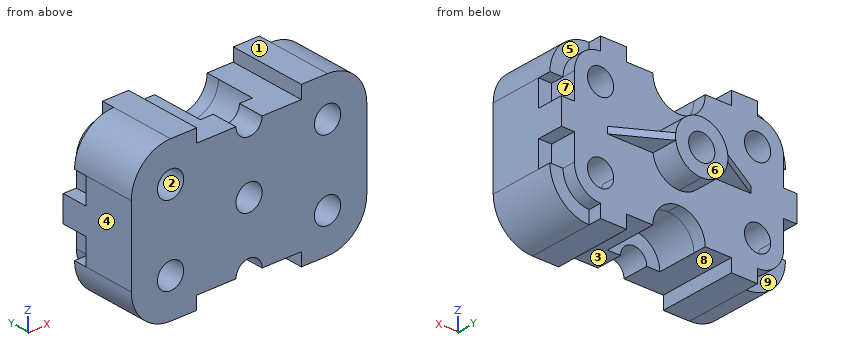
```python
from build123d import *

# Parameters (mm, degrees)
SKETCH1_W           = 180
SKETCH1_H           = 120
BOSS_EXTRUDE2_DEPTH = 80
CUT_EXTRUDE1_DEPTH  = 150
CUT_EXTRUDE2_DEPTH  = 150
SKETCH4_R           = 10
CUT_EXTRUDE3_DEPTH  = 150
CUT_EXTRUDE4_DEPTH  = 60
CUT_EXTRUDE5_DEPTH  = 60
SKETCH7_R           = 10
CUT_EXTRUDE7_DEPTH  = 139
SKETCH8_W           = 80
SKETCH8_H           = 10
CUT_EXTRUDE8_DEPTH  = 139
BOSS_EXTRUDE3_DEPTH = 60
CUT_EXTRUDE9_DEPTH  = 256
CUT_EXTRUDE10_DEPTH = 60
CUT_EXTRUDE11_DEPTH = 60
SKETCH13_W          = 40
SKETCH13_H          = 20
SKETCH13_W_2        = 20
SKETCH13_H_2        = 10
CUT_EXTRUDE12_DEPTH = 209
CUT_EXTRUDE13_DEPTH = 20
CUT_EXTRUDE14_DEPTH = 10
CUT_EXTRUDE15_DEPTH = 10
CUT_EXTRUDE16_DEPTH = 10
CUT_EXTRUDE17_DEPTH = 10
BOSS_EXTRUDE4_DEPTH = 10
BOSS_EXTRUDE5_DEPTH = 10
SKETCH21_W          = 10
SKETCH21_H          = 20
CUT_EXTRUDE20_DEPTH = 20
SKETCH22_W          = 35
SKETCH22_H          = 5
BOSS_EXTRUDE9_DEPTH = 19.999
CUT_EXTRUDE21_DEPTH = 10


with BuildPart() as part:
    # Sketch1 → Boss-Extrude2 (new body)
    with BuildSketch(Plane(origin=(0, 0, 0), x_dir=(1, 0, 0), z_dir=(0, 1, 0))):
        with Locations((90, 60)):
            Rectangle(SKETCH1_W, SKETCH1_H)
    extrude(amount=BOSS_EXTRUDE2_DEPTH)

    # Sketch2 → Cut-Extrude1 (cut)
    with BuildSketch(Plane(origin=(0, 0, 0), x_dir=(1, 0, 0), z_dir=(0, 1, 0))):
        with BuildLine():
            ThreePointArc((30, 0), (8.786796564, 8.786796564), (0, 30))
            Line((0, 30), (0, 0))
            Line((0, 0), (30, 0))
        make_face()
        with BuildLine():
            Line((180, 0), (180, 30))
            ThreePointArc((180, 30), (171.213203436, 8.786796564), (150, 0))
            Line((150, 0), (180, 0))
        make_face()
        with BuildLine():
            Line((180, 120), (150, 120))
            ThreePointArc((150, 120), (171.213203436, 111.213203436), (180, 90))
            Line((180, 90), (180, 120))
        make_face()
        with BuildLine():
            Line((0, 120), (30, 120))
            ThreePointArc((30, 120), (8.786796564, 111.213203436), (0, 90))
            Line((0, 90), (0, 120))
        make_face()
    extrude(amount=CUT_EXTRUDE1_DEPTH, mode=Mode.SUBTRACT)

    # Sketch3 → Cut-Extrude2 (cut)
    with BuildSketch(Plane(origin=(0, 0, 0), x_dir=(1, 0, 0), z_dir=(0, 1, 0))):
        with BuildLine():
            Line((80, 120), (100, 120))
            ThreePointArc((100, 120), (90, 110), (80, 120))
        make_face()
        with BuildLine():
            Line((80, 0), (100, 0))
            ThreePointArc((100, 0), (90, 10), (80, 0))
        make_face()
    extrude(amount=CUT_EXTRUDE2_DEPTH, mode=Mode.SUBTRACT)

    # Sketch4 → Cut-Extrude3 (cut)
    with BuildSketch(Plane(origin=(0, 80, 0), x_dir=(1, 0, 0), z_dir=(0, 1, 0))):
        with Locations(Location((30, 90, 0), (0, 0, 270))):
            Circle(SKETCH4_R)
        with Locations(Location((150, 90, 0), (0, 0, 270))):
            Circle(SKETCH4_R)
        with Locations(Location((150, 30, 0), (0, 0, 270))):
            Circle(SKETCH4_R)
        with Locations(Location((30, 30, 0), (0, 0, 270))):
            Circle(SKETCH4_R)
    extrude(amount=-CUT_EXTRUDE3_DEPTH, mode=Mode.SUBTRACT)

    # Sketch5 → Cut-Extrude4 (cut)
    with BuildSketch(Plane(origin=(0, 80, 0), x_dir=(1, 0, 0), z_dir=(0, 1, 0))):
        with BuildLine():
            Line((70, 120), (80, 120))
            ThreePointArc((80, 120), (90, 110), (100, 120))
            Line((100, 120), (110, 120))
            ThreePointArc((110, 120), (90, 100), (70, 120))
        make_face()
    extrude(amount=-CUT_EXTRUDE4_DEPTH, mode=Mode.SUBTRACT)

    # Sketch6 → Cut-Extrude5 (cut)
    with BuildSketch(Plane(origin=(0, 80, 0), x_dir=(1, 0, 0), z_dir=(0, 1, 0))):
        with BuildLine():
            ThreePointArc((110, 0), (90, 20), (70, 0))
            Line((70, 0), (80, 0))
            ThreePointArc((80, 0), (90, 10), (100, 0))
            Line((100, 0), (110, 0))
        make_face()
    extrude(amount=-CUT_EXTRUDE5_DEPTH, mode=Mode.SUBTRACT)

    # Sketch7 → Cut-Extrude7 (cut)
    with BuildSketch(Plane(origin=(0, 80, 0), x_dir=(1, 0, 0), z_dir=(0, 1, 0))):
        with Locations(Location((90, 60, 0), (0, 0, 270))):
            Circle(SKETCH7_R)
    extrude(amount=-CUT_EXTRUDE7_DEPTH, mode=Mode.SUBTRACT)

    # Sketch8 → Cut-Extrude8 (cut)
    with BuildSketch(Plane(origin=(0, 80, 0), x_dir=(1, 0, 0), z_dir=(0, 1, 0))):
        with Locations((90, 115)):
            Rectangle(SKETCH8_W, SKETCH8_H)
        with Locations((90, 5)):
            Rectangle(SKETCH8_W, SKETCH8_H)
    extrude(amount=-CUT_EXTRUDE8_DEPTH, mode=Mode.SUBTRACT)

    # Sketch9 → Boss-Extrude3 (add)
    with BuildSketch(Plane(origin=(0, 20, 0), x_dir=(1, 0, 0), z_dir=(0, 1, 0))):
        with BuildLine():
            Line((72.679491924, 110), (107.320508076, 110))
            ThreePointArc((107.320508076, 110), (90, 100), (72.679491924, 110))
        make_face()
        with BuildLine():
            Line((72.679491924, 10), (107.320508076, 10))
            ThreePointArc((107.320508076, 10), (90, 20), (72.679491924, 10))
        make_face()
    extrude(amount=BOSS_EXTRUDE3_DEPTH)

    # Sketch10 → Cut-Extrude9 (cut)
    with BuildSketch(Plane(origin=(0, 80, 0), x_dir=(1, 0, 0), z_dir=(0, 1, 0))):
        with BuildLine():
            Line((80, 110), (100, 110))
            ThreePointArc((100, 110), (90, 100), (80, 110))
        make_face()
        with BuildLine():
            Line((80, 10), (100, 10))
            ThreePointArc((100, 10), (90, 20), (80, 10))
        make_face()
    extrude(amount=-CUT_EXTRUDE9_DEPTH, mode=Mode.SUBTRACT)

    # Sketch11 → Cut-Extrude10 (cut)
    with BuildSketch(Plane(origin=(0, 80, 0), x_dir=(1, 0, 0), z_dir=(0, 1, 0))):
        with BuildLine():
            Line((80, 110), (70, 110))
            ThreePointArc((70, 110), (90, 90), (110, 110))
            Line((110, 110), (100, 110))
            ThreePointArc((100, 110), (90, 100), (80, 110))
        make_face()
    extrude(amount=-CUT_EXTRUDE10_DEPTH, mode=Mode.SUBTRACT)

    # Sketch12 → Cut-Extrude11 (cut)
    with BuildSketch(Plane(origin=(0, 80, 0), x_dir=(1, 0, 0), z_dir=(0, 1, 0))):
        with BuildLine():
            ThreePointArc((110, 10), (90, 30), (70, 10))
            Line((70, 10), (80, 10))
            ThreePointArc((80, 10), (90, 20), (100, 10))
            Line((100, 10), (110, 10))
        make_face()
    extrude(amount=-CUT_EXTRUDE11_DEPTH, mode=Mode.SUBTRACT)

    # Sketch13 → Cut-Extrude12 (cut)
    with BuildSketch(Plane(origin=(0, 0, 0), x_dir=(0, 0, -1), z_dir=(1, 0, 0))):
        with Locations((100, 70)):
            Rectangle(SKETCH13_W, SKETCH13_H)
        with Locations((100, 55)):
            Rectangle(SKETCH13_W_2, SKETCH13_H_2)
        with Locations((20, 70)):
            Rectangle(SKETCH13_W, SKETCH13_H)
        with Locations((20, 55)):
            Rectangle(SKETCH13_W_2, SKETCH13_H_2)
    extrude(amount=CUT_EXTRUDE12_DEPTH, mode=Mode.SUBTRACT)

    # Sketch14 → Cut-Extrude13 (cut)
    with BuildSketch(Plane(origin=(0, 80, 0), x_dir=(1, 0, 0), z_dir=(0, 1, 0))):
        with BuildLine():
            Line((90, 80), (0, 80))
            Line((0, 80), (0, 40))
            Line((0, 40), (90, 40))
            ThreePointArc((90, 40), (70, 60), (90, 80))
        make_face()
        with BuildLine():
            Line((180, 80), (90, 80))
            ThreePointArc((90, 80), (104.142135624, 74.142135624), (110, 60))
            ThreePointArc((110, 60), (104.142135624, 45.857864376), (90, 40))
            Line((90, 40), (180, 40))
            Line((180, 40), (180, 80))
        make_face()
    extrude(amount=-CUT_EXTRUDE13_DEPTH, mode=Mode.SUBTRACT)

    # Sketch15 → Cut-Extrude14 (cut)
    with BuildSketch(Plane(origin=(0, 60, 0), x_dir=(1, 0, 0), z_dir=(0, 1, 0))):
        with BuildLine():
            Line((7.639320225, 110), (30, 110))
            Line((30, 110), (30, 120))
            ThreePointArc((30, 120), (17.752551286, 117.386127875), (7.639320225, 110))
        make_face()
    extrude(amount=-CUT_EXTRUDE14_DEPTH, mode=Mode.SUBTRACT)

    # Sketch16 → Cut-Extrude15 (cut)
    with BuildSketch(Plane(origin=(0, 60, 0), x_dir=(1, 0, 0), z_dir=(0, 1, 0))):
        with BuildLine():
            ThreePointArc((7.639320225, 10), (17.752551286, 2.613872125), (30, 0))
            Line((30, 0), (30, 10))
            Line((30, 10), (7.639320225, 10))
        make_face()
    extrude(amount=-CUT_EXTRUDE15_DEPTH, mode=Mode.SUBTRACT)

    # Sketch17 → Cut-Extrude16 (cut)
    with BuildSketch(Plane(origin=(0, 60, 0), x_dir=(1, 0, 0), z_dir=(0, 1, 0))):
        with BuildLine():
            Line((150, 10), (150, 0))
            ThreePointArc((150, 0), (162.247448714, 2.613872125), (172.360679775, 10))
            Line((172.360679775, 10), (150, 10))
        make_face()
    extrude(amount=-CUT_EXTRUDE16_DEPTH, mode=Mode.SUBTRACT)

    # Sketch18 → Cut-Extrude17 (cut)
    with BuildSketch(Plane(origin=(0, 60, 0), x_dir=(1, 0, 0), z_dir=(0, 1, 0))):
        with BuildLine():
            ThreePointArc((172.360679775, 110), (162.247448714, 117.386127875), (150, 120))
            Line((150, 120), (150, 110))
            Line((150, 110), (172.360679775, 110))
        make_face()
    extrude(amount=-CUT_EXTRUDE17_DEPTH, mode=Mode.SUBTRACT)

    # Sketch19 → Boss-Extrude4 (add)
    with BuildSketch(Plane(origin=(0, 50, 0), x_dir=(1, 0, 0), z_dir=(0, 1, 0))):
        with BuildLine():
            Line((40, 90), (90, 90))
            ThreePointArc((90, 90), (75.857864376, 95.857864376), (70, 110))
            Line((70, 110), (30, 110))
            ThreePointArc((30, 110), (15.857864376, 104.142135624), (10, 90))
            Line((10, 90), (20, 90))
            ThreePointArc((20, 90), (30, 100), (40, 90))
        make_face()
        with BuildLine():
            ThreePointArc((170, 90), (164.142135624, 104.142135624), (150, 110))
            Line((150, 110), (130, 110))
            Line((130, 110), (110, 110))
            ThreePointArc((110, 110), (104.142135624, 95.857864376), (90, 90))
            Line((90, 90), (140, 90))
            ThreePointArc((140, 90), (150, 100), (160, 90))
            Line((160, 90), (170, 90))
        make_face()
    extrude(amount=BOSS_EXTRUDE4_DEPTH)

    # Sketch20 → Boss-Extrude5 (add)
    with BuildSketch(Plane(origin=(0, 50, 0), x_dir=(1, 0, 0), z_dir=(0, 1, 0))):
        with BuildLine():
            Line((20, 30), (10, 30))
            ThreePointArc((10, 30), (15.857864376, 15.857864376), (30, 10))
            Line((30, 10), (50, 10))
            Line((50, 10), (70, 10))
            ThreePointArc((70, 10), (75.857864376, 24.142135624), (90, 30))
            Line((90, 30), (40, 30))
            ThreePointArc((40, 30), (30, 20), (20, 30))
        make_face()
        with BuildLine():
            Line((140, 30), (90, 30))
            ThreePointArc((90, 30), (104.142135624, 24.142135624), (110, 10))
            Line((110, 10), (130, 10))
            Line((130, 10), (150, 10))
            ThreePointArc((150, 10), (164.142135624, 15.857864376), (170, 30))
            Line((170, 30), (160, 30))
            ThreePointArc((160, 30), (150, 20), (140, 30))
        make_face()
    extrude(amount=BOSS_EXTRUDE5_DEPTH)

    # Sketch21 → Cut-Extrude20 (cut)
    with BuildSketch(Plane(origin=(0, 60, 0), x_dir=(1, 0, 0), z_dir=(0, 1, 0))):
        with Locations((5, 80)):
            Rectangle(SKETCH21_W, SKETCH21_H)
        with Locations((5, 40)):
            Rectangle(SKETCH21_W, SKETCH21_H)
        with Locations((175, 80)):
            Rectangle(SKETCH21_W, SKETCH21_H)
        with Locations((175, 40)):
            Rectangle(SKETCH21_W, SKETCH21_H)
    extrude(amount=-CUT_EXTRUDE20_DEPTH, mode=Mode.SUBTRACT)

    # Sketch22 → Boss-Extrude9 (add)
    with BuildSketch(Plane(origin=(0, 60, 0), x_dir=(1, 0, 0), z_dir=(0, 1, 0))):
        with BuildLine():
            Line((70.156865167, 62.5), (35.156865167, 62.5))
            Line((35.156865167, 62.5), (35.156865167, 57.5))
            Line((35.156865167, 57.5), (70.156865167, 57.5))
            ThreePointArc((70.156865167, 57.5), (70, 60), (70.156865167, 62.5))
        make_face()
        with Locations((127.343134833, 60)):
            Rectangle(SKETCH22_W, SKETCH22_H)
    extrude(amount=BOSS_EXTRUDE9_DEPTH)

    # Sketch23 → Cut-Extrude21 (cut)
    with BuildSketch(Plane.XY.offset(-57.5)):
        Polygon((35.156865167, 60), (70.156865167, 79.999), (35.156865167, 79.999), align=None)
        Polygon((109.843134833, 79.999), (144.843134833, 60), (144.843134833, 79.999), align=None)
    extrude(amount=-CUT_EXTRUDE21_DEPTH, mode=Mode.SUBTRACT)


solid = part.part
```
Verification items for the finished model (mm, model axes). Face numbers are marked on the shaded views. A direction names the side the tool comes from. Coordinates: 2 decimals unless noted, no trailing zeros. Loops run counter-clockwise (first coordinate to the right, second up) from the corner with the lowest first, then second, coordinate; pieces in that order, holes last. Notation, with made-up numbers: (77.25, -11) -> (124.25, -11) arc R8 ccw to (124.25, -4) -> close; hole circle Ø6 at (-8, 60). An arc over 180 degrees is marked (long way). Put each result on its own line as item: value.
1. Tool access check on the marked faces 5, 6, 7, 8 and 9. Record the directions out of +Z, -Z, +X, -X, +Y, -Y that give a thin tool (end or side, any length) a straight path to the whole face; none if there is none.
Result set:
face 5: +Z, +X, +Y
face 6: +Z, -Z, +X, -X, +Y
face 7: +X, +Y
face 8: -Z, +Y, -Y
face 9: -Z, -X, +Y
2. Section check A-A, the plane z = -16. Record the boundary of the cut face in (x, y), then the cut area to 3 significant figures.
Result set:
outline: (3.47, 0) -> (82, 0) -> (82, 20) -> (70.92, 20) -> (70.92, 60) -> (15.72, 60) -> (15.72, 50) -> (3.47, 50) -> close; (98, 0) -> (176.53, 0) -> (176.53, 50) -> (164.28, 50) -> (164.28, 60) -> (109.08, 60) -> (109.08, 20) -> (98, 20) -> close
area: 8,290 mm^2
3. Thickness scan on line 1 (Z direction, x = 150, y = 32); line 2 (X direction, y = 19, z = -90); line 3 (X direction, y = 59, z = -94.5). Record the ranges inside material, lowest first.
Result set:
line 1: z = -120 to -100, -80 to -40, -20 to 0
line 2: x = 0 to 20, 40 to 140, 160 to 180
line 3: x = 10.51 to 21.07, 38.93 to 77.36, 102.64 to 141.07, 158.93 to 169.49
4. Gauge pin test, flat ends, axial feed: P1, Ø22, axis at x = 80, z = -100.5, coming from the +Y side; P2, Ø15, axis at x = 60, y = 44, coming from the -Z side; P3, Ø2, axis at x = 155, y = 14, coming from the +Z side. Record the tip position at first contact, or that the pin passes through.
Result set:
P1: stops at y = 60
P2: stops at z = -110
P3: stops at z = -0.27
5. Mould release check, pull along Z, two halves, no side actions. Record for the marked faces 1, 2, 3 and 4: pulls with the +Z half, pulls with the -Z half, needs draft (parallel to the pull), parting line crosses it, or undercut.
Result set:
face 1: pulls with the +Z half
face 2: undercut
face 3: pulls with the -Z half
face 4: needs draft
6. Section check C-C, the plane x = 95. Record the boundary of the cut face in (y, z).
Result set:
outline: (0, -101.34) -> (20, -101.34) -> (20, -90.64) -> (60, -90.64) -> (60, -79.36) -> (80, -79.36) -> (80, -68.66) -> (0, -68.66) -> close; (0, -51.34) -> (80, -51.34) -> (80, -40.64) -> (60, -40.64) -> (60, -29.36) -> (20, -29.36) -> (20, -18.66) -> (0, -18.66) -> close
7. Section check B-B, the plane y = 15. Record the boundary of the cut face in (x, z).
Result set:
outline: (0, -90) arc R30 ccw to (30, -120) -> (50, -120) -> (50, -110) -> (80, -110) arc R10 cw to (100, -110) -> (130, -110) -> (130, -120) -> (150, -120) arc R30 ccw to (180, -90) -> (180, -30) arc R30 ccw to (150, 0) -> (130, 0) -> (130, -10) -> (100, -10) arc R10 cw to (80, -10) -> (50, -10) -> (50, 0) -> (30, 0) arc R30 ccw to (0, -30) -> close; hole circle Ø20 at (30, -90); hole circle Ø20 at (30, -30); hole circle Ø20 at (90, -60); hole circle Ø20 at (150, -90); hole circle Ø20 at (150, -30)
8. Section check D-D, the plane z = -88. Record the boundary of the cut face in (x, y), then the cut area to 3 significant figures.
Result set:
outline: (0, 0) -> (20.2, 0) -> (20.2, 60) -> (10, 60) -> (10, 40) -> (0, 40) -> close; (39.8, 0) -> (140.2, 0) -> (140.2, 60) -> (39.8, 60) -> close; (159.8, 0) -> (180, 0) -> (180, 40) -> (170, 40) -> (170, 60) -> (159.8, 60) -> close
area: 8,050 mm^2
